from build123d import *

# Parameters (mm, degrees)
F0_W     = 123.0850573922
F0_H     = 25
F0_R     = 2.5
F1_DEPTH = 40
F2_DEPTH = 40
F3_DEPTH = 5
F4_R     = 2.5


# Not quite as in the source:
# - a feature names something its author has since deleted; it is built from what else it names


with BuildPart() as f1:
    # F0 (on Top) → F1 (new body)
    with BuildSketch(Plane.XY):
        with Locations((18.6507174147, 3.4210662183)):
            Rectangle(F0_W, F0_H)
        with Locations((-35.3918112814, -1.5789337817)):
            Circle(F0_R, mode=Mode.SUBTRACT)
        with Locations((-27.0588112814, -1.5789337817)):
            Circle(F0_R, mode=Mode.SUBTRACT)
        with Locations((-18.7258112814, -1.5789337817)):
            Circle(F0_R, mode=Mode.SUBTRACT)
        with Locations((-10.3928112814, -1.5789337817)):
            Circle(F0_R, mode=Mode.SUBTRACT)
        with Locations((-2.0598112814, -1.5789337817)):
            Circle(F0_R, mode=Mode.SUBTRACT)
        with Locations((6.2731887186, -1.5789337817)):
            Circle(F0_R, mode=Mode.SUBTRACT)
        with Locations((14.6061887186, -1.5789337817)):
            Circle(F0_R, mode=Mode.SUBTRACT)
        with Locations((22.9391887186, -1.5789337817)):
            Circle(F0_R, mode=Mode.SUBTRACT)
        with Locations((31.2721887186, -1.5789337817)):
            Circle(F0_R, mode=Mode.SUBTRACT)
        with Locations((39.6051887186, -1.5789337817)):
            Circle(F0_R, mode=Mode.SUBTRACT)
        with Locations((47.9381887186, -1.5789337817)):
            Circle(F0_R, mode=Mode.SUBTRACT)
        with Locations((56.2711887186, -1.5789337817)):
            Circle(F0_R, mode=Mode.SUBTRACT)
        with Locations((64.6041887186, -1.5789337817)):
            Circle(F0_R, mode=Mode.SUBTRACT)
        with Locations((72.9371887186, -1.5789337817)):
            Circle(F0_R, mode=Mode.SUBTRACT)
        with Locations((-35.3918112814, 8.4210662183)):
            Circle(F0_R, mode=Mode.SUBTRACT)
        with Locations((-27.0588112814, 8.4210662183)):
            Circle(F0_R, mode=Mode.SUBTRACT)
        with Locations((-18.7258112814, 8.4210662183)):
            Circle(F0_R, mode=Mode.SUBTRACT)
        with Locations((-10.3928112814, 8.4210662183)):
            Circle(F0_R, mode=Mode.SUBTRACT)
        with Locations((-2.0598112814, 8.4210662183)):
            Circle(F0_R, mode=Mode.SUBTRACT)
        with Locations((6.2731887186, 8.4210662183)):
            Circle(F0_R, mode=Mode.SUBTRACT)
        with Locations((14.6061887186, 8.4210662183)):
            Circle(F0_R, mode=Mode.SUBTRACT)
        with Locations((22.9391887186, 8.4210662183)):
            Circle(F0_R, mode=Mode.SUBTRACT)
        with Locations((31.2721887186, 8.4210662183)):
            Circle(F0_R, mode=Mode.SUBTRACT)
        with Locations((39.6051887186, 8.4210662183)):
            Circle(F0_R, mode=Mode.SUBTRACT)
        with Locations((47.9381887186, 8.4210662183)):
            Circle(F0_R, mode=Mode.SUBTRACT)
        with Locations((56.2711887186, 8.4210662183)):
            Circle(F0_R, mode=Mode.SUBTRACT)
        with Locations((64.6041887186, 8.4210662183)):
            Circle(F0_R, mode=Mode.SUBTRACT)
        with Locations((72.9371887186, 8.4210662183)):
            Circle(F0_R, mode=Mode.SUBTRACT)
        with Locations((-35.3918112814, 8.4210662183)):
            Circle(F0_R)
        with Locations((-27.0588112814, 8.4210662183)):
            Circle(F0_R)
        with Locations((-27.0588112814, -1.5789337817)):
            Circle(F0_R)
        with Locations((-35.3918112814, -1.5789337817)):
            Circle(F0_R)
    extrude(amount=-F1_DEPTH)

    # F0 (on Top) → F2 (cut)
    with BuildSketch(Plane.XY):
        with Locations((-35.3918112814, 8.4210662183)):
            Circle(F0_R)
        with Locations((-27.0588112814, 8.4210662183)):
            Circle(F0_R)
        with Locations((-18.7258112814, 8.4210662183)):
            Circle(F0_R)
        with Locations((-10.3928112814, 8.4210662183)):
            Circle(F0_R)
        with Locations((-2.0598112814, 8.4210662183)):
            Circle(F0_R)
        with Locations((6.2731887186, 8.4210662183)):
            Circle(F0_R)
        with Locations((14.6061887186, 8.4210662183)):
            Circle(F0_R)
        with Locations((22.9391887186, 8.4210662183)):
            Circle(F0_R)
        with Locations((31.2721887186, 8.4210662183)):
            Circle(F0_R)
        with Locations((39.6051887186, 8.4210662183)):
            Circle(F0_R)
        with Locations((47.9381887186, 8.4210662183)):
            Circle(F0_R)
        with Locations((56.2711887186, 8.4210662183)):
            Circle(F0_R)
        with Locations((64.6041887186, 8.4210662183)):
            Circle(F0_R)
        with Locations((72.9371887186, 8.4210662183)):
            Circle(F0_R)
    extrude(amount=-F2_DEPTH, mode=Mode.SUBTRACT)

    # F0 (on Top) → F3 (cut)
    with BuildSketch(Plane.XY):
        with Locations((-35.3918112814, -1.5789337817)):
            Circle(F0_R)
        with Locations((-27.0588112814, -1.5789337817)):
            Circle(F0_R)
    extrude(amount=-F3_DEPTH, mode=Mode.SUBTRACT)

    # F4
    f4_edges = [f1.edges().sort_by_distance(p)[0] for p in [
        (-37.891811, -1.578934, -5),
        (-29.558811, -1.578934, -5),
    ]]
    fillet(f4_edges, radius=F4_R)


solid = f1.part
Input: part model. Units: mm. Frame: model coordinates. A direction names the side the tool comes from. Round coordinates to 2 decimals unless told otherwise and drop trailing zeros. Order: outer loops, then holes, each group sorted by start corner. A loop starts at its lowest first (then second) coordinate and runs counter-clockwise, first axis right, second up.
1. Cut plane B-B, the plane z = -33. State how many separate pieces and enclosed holes the cut face has, then the cut area to 3 significant figures.
The answers:
separate pieces: 1
enclosed holes: 26
area: 2,570 mm2
2. Cut plane A-A, the plane x = -1.5. Output: boundary loops of the cut face in (y, z).
The answers:
outline: (-9.08, -40) - (-4.02, -40) - (-4.02, 0) - (-9.08, 0) - close; (0.86, -40) - (5.98, -40) - (5.98, 0) - (0.86, 0) - close; (10.86, -40) - (15.92, -40) - (15.92, 0) - (10.86, 0) - close
3. Mould query, pull axis Y, two halves, no side actions, for faces 1 (the face through (18, 4, 0)), 2 (the face through (37.62, 6.9, -19.72)), 3 (the face through (18, -9.079, -20)). Classes: released by +Y, released by -Y, zero draft, split by the parting line, or undercut.
The answers:
face 1: zero draft
face 2: undercut
face 3: released by -Y
4. Material intervals for line 1 (Y direction, x = 56, z = -14.5); line 2 (Y direction, x = 47, z = -30); line 3 (Y direction, x = -26, z = -22), sorted ascending.
The answers:
line 1: y = -9.08 to -4.06, 0.91 to 5.94, 10.91 to 15.92
line 2: y = -9.08 to -3.9, 0.74 to 6.1, 10.74 to 15.92
line 3: y = -9.08 to 6.16, 10.69 to 15.92
5. Pin query (flat end, axial travel): P1, Ø4, axis at x = 56.27, y = 8.42, coming from the -Z side; P2, Ø6.5, axis at x = 64.6, y = 8.42, coming from the +Z side. Return the tip coordinate at first contact, or that it passes through.
The answers:
P1: passes through
P2: stops at z = 0
6. Set-up query: faces 4 (the face through (7.427, 6.203, -19.72)), 5 (the face through (-33.082, -2.536, -1.232)). Return all of +Z, -Z, +X, -X, +Y, -Y with unobstructed straight access to the full face (end or side cutting, diameter ignored); none if empty.
The answers:
face 4: +Z, -Z
face 5: +Z
7. Cut plane C-C, the plane x = 30. Output: boundary loops of the cut face in (y, z), then the cut area to 3 significant figures.
The answers:
outline: (-9.08, -40) - (-3.73, -40) - (-3.73, 0) - (-9.08, 0) - close; (0.57, -40) - (6.27, -40) - (6.27, 0) - (0.57, 0) - close; (10.57, -40) - (15.92, -40) - (15.92, 0) - (10.57, 0) - close
area: 656 mm2
